from build123d import *

# Parameters (mm, degrees)
BOSS_EXTRUDE1_DEPTH = 38.1
SKETCH2_W           = 209.55
SKETCH2_H           = 38.1
BOSS_EXTRUDE2_DEPTH = 9.525
SKETCH3_W           = 20.32
SKETCH3_H           = 3.175
SKETCH3_H_2         = 6.35
SKETCH3_H_3         = 9.525
SKETCH3_H_4         = 12.7
SKETCH3_H_5         = 15.875
SKETCH3_H_6         = 19.05
SKETCH3_H_7         = 22.225
SKETCH3_H_8         = 25.4
CUT_EXTRUDE1_DEPTH  = 123.141181515
CHAMFER1_SIZE       = 25.4
CHAMFER2_SIZE       = 25.4
FILLET1_R           = 1.27
FILLET2_R           = 5.08


with BuildPart() as part:
    # Sketch1 → Boss-Extrude1 (new, symmetric)
    with BuildSketch(Plane.XY):
        Polygon((-105.823993484, 0), (103.726006516, 0), (103.726006516, 12.7), (-105.823993484, 25.4), align=None)
    extrude(amount=BOSS_EXTRUDE1_DEPTH, both=True)

    # Sketch2 → Boss-Extrude2 (add)
    with BuildSketch(Plane(origin=(0, 0, -38.1), x_dir=(-1, 0, 0), z_dir=(0, 0, -1))):
        with Locations((1.048993484, 19.05)):
            Rectangle(SKETCH2_W, SKETCH2_H)
    boss_extrude2 = extrude(amount=BOSS_EXTRUDE2_DEPTH)

    # Mirror1: Boss-Extrude2 across plane
    add(boss_extrude2.mirror(Plane.XY))

    # Sketch3 → Cut-Extrude1 (cut, through all)
    with BuildSketch(Plane.XZ):
        with Locations((-89.313993484, 0)):
            Rectangle(SKETCH3_W, SKETCH3_H)
        with Locations((-63.151993484, 0)):
            Rectangle(SKETCH3_W, SKETCH3_H_2)
        with Locations((-36.989993484, 0)):
            Rectangle(SKETCH3_W, SKETCH3_H_3)
        with Locations((-10.827993484, 0)):
            Rectangle(SKETCH3_W, SKETCH3_H_4)
        with Locations((15.334006516, 0)):
            Rectangle(SKETCH3_W, SKETCH3_H_5)
        with Locations((41.496006516, 0)):
            Rectangle(SKETCH3_W, SKETCH3_H_6)
        with Locations((67.658006516, 0)):
            Rectangle(SKETCH3_W, SKETCH3_H_7)
        with Locations((93.566006516, 0)):
            Rectangle(SKETCH3_W, SKETCH3_H_8)
    extrude(amount=-CUT_EXTRUDE1_DEPTH, mode=Mode.SUBTRACT)

    # Chamfer1
    # the kernel refuses this chamfer: 25.4 mm, written as the material it adds along each edge
    with BuildSketch(Plane(origin=(168.92711924, 8.748417411, 38.1), x_dir=(0.060472188242602316, 0.9977911060029382, 0.02749587661058647), z_dir=(-0.9981684966311909, 0.06049506040189036, 0))) as chamfer1_piece_1_section:
        Polygon((CHAMFER1_SIZE * 0.999621916911, CHAMFER1_SIZE * 0.0274958766106), (-CHAMFER1_SIZE * 0.0274958766106, CHAMFER1_SIZE * 0.999621916911), (0, 0), align=None)
    chamfer1_piece_1 = extrude(amount=340.575991525, mode=Mode.PRIVATE)
    chamfer1_piece_1 = split(chamfer1_piece_1, bisect_by=Plane(origin=(103.726006516, 21.644739683, 29.711789503), z_dir=(-1, 0, 0)), keep=Keep.TOP, mode=Mode.PRIVATE)
    chamfer1_piece_1 = split(chamfer1_piece_1, bisect_by=Plane(origin=(93.576497018, 21.644739683, 12.7), z_dir=(0, 0, 1)), keep=Keep.TOP, mode=Mode.PRIVATE)
    chamfer1_piece_1 = split(chamfer1_piece_1, bisect_by=Plane(origin=(83.406006516, 21.644739683, 29.711789503), z_dir=(1, 0, 0)), keep=Keep.TOP, mode=Mode.PRIVATE)
    chamfer1_piece_1 = split(chamfer1_piece_1, bisect_by=Plane(origin=(93.576497018, 38.1, 29.711789503), z_dir=(0, -1, 0)), keep=Keep.TOP, mode=Mode.PRIVATE)
    add(chamfer1_piece_1)
    with BuildSketch(Plane(origin=(168.92711924, 8.748417411, 38.1), x_dir=(0.060472188242602316, 0.9977911060029382, 0.02749587661058647), z_dir=(-0.9981684966311909, 0.06049506040189036, 0))) as chamfer1_piece_2_section:
        Polygon((CHAMFER1_SIZE * 0.999621916911, CHAMFER1_SIZE * 0.0274958766106), (-CHAMFER1_SIZE * 0.0274958766106, CHAMFER1_SIZE * 0.999621916911), (0, 0), align=None)
    chamfer1_piece_2 = extrude(amount=340.575991525, mode=Mode.PRIVATE)
    chamfer1_piece_2 = split(chamfer1_piece_2, bisect_by=Plane(origin=(-105.823993484, 26.508792165, 29.076634432), z_dir=(1, 0, 0)), keep=Keep.TOP, mode=Mode.PRIVATE)
    chamfer1_piece_2 = split(chamfer1_piece_2, bisect_by=Plane(origin=(-6.816832876, 26.508792165, 12.7), z_dir=(0, 0, 1)), keep=Keep.TOP, mode=Mode.PRIVATE)
    chamfer1_piece_2 = split(chamfer1_piece_2, bisect_by=Plane(origin=(83.406006516, 26.508792165, 29.076634432), z_dir=(-1, 0, 0)), keep=Keep.TOP, mode=Mode.PRIVATE)
    chamfer1_piece_2 = split(chamfer1_piece_2, bisect_by=Plane(origin=(-6.816832876, 38.1, 29.076634432), z_dir=(0, -1, 0)), keep=Keep.TOP, mode=Mode.PRIVATE)
    add(chamfer1_piece_2)

    # Chamfer2
    # the kernel refuses this chamfer: 25.4 mm, written as the material it adds along each edge
    with BuildSketch(Plane(origin=(168.92711924, 8.748417411, -38.1), x_dir=(0.060472188242602316, 0.9977911060029382, -0.02749587661058647), z_dir=(-0.9981684966311909, 0.06049506040189036, 0))) as chamfer2_piece_1_section:
        Polygon((CHAMFER2_SIZE * 0.999621916911, -CHAMFER2_SIZE * 0.0274958766106), (-CHAMFER2_SIZE * 0.0274958766106, -CHAMFER2_SIZE * 0.999621916911), (0, 0), align=None)
    chamfer2_piece_1 = extrude(amount=340.575991525, mode=Mode.PRIVATE)
    chamfer2_piece_1 = split(chamfer2_piece_1, bisect_by=Plane(origin=(93.576497018, 38.1, -29.711789503), z_dir=(0, -1, 0)), keep=Keep.TOP, mode=Mode.PRIVATE)
    chamfer2_piece_1 = split(chamfer2_piece_1, bisect_by=Plane(origin=(103.726006516, 21.644739683, -29.711789503), z_dir=(-1, 0, 0)), keep=Keep.TOP, mode=Mode.PRIVATE)
    chamfer2_piece_1 = split(chamfer2_piece_1, bisect_by=Plane(origin=(93.576497018, 21.644739683, -12.7), z_dir=(0, 0, -1)), keep=Keep.TOP, mode=Mode.PRIVATE)
    chamfer2_piece_1 = split(chamfer2_piece_1, bisect_by=Plane(origin=(83.406006516, 21.644739683, -29.711789503), z_dir=(1, 0, 0)), keep=Keep.TOP, mode=Mode.PRIVATE)
    add(chamfer2_piece_1)
    with BuildSketch(Plane(origin=(168.92711924, 8.748417411, -38.1), x_dir=(0.060472188242602316, 0.9977911060029382, -0.02749587661058647), z_dir=(-0.9981684966311909, 0.06049506040189036, 0))) as chamfer2_piece_2_section:
        Polygon((CHAMFER2_SIZE * 0.999621916911, -CHAMFER2_SIZE * 0.0274958766106), (-CHAMFER2_SIZE * 0.0274958766106, -CHAMFER2_SIZE * 0.999621916911), (0, 0), align=None)
    chamfer2_piece_2 = extrude(amount=340.575991525, mode=Mode.PRIVATE)
    chamfer2_piece_2 = split(chamfer2_piece_2, bisect_by=Plane(origin=(-105.823993484, 26.508792165, -29.076634432), z_dir=(1, 0, 0)), keep=Keep.TOP, mode=Mode.PRIVATE)
    chamfer2_piece_2 = split(chamfer2_piece_2, bisect_by=Plane(origin=(-6.816832876, 38.1, -29.076634432), z_dir=(0, -1, 0)), keep=Keep.TOP, mode=Mode.PRIVATE)
    chamfer2_piece_2 = split(chamfer2_piece_2, bisect_by=Plane(origin=(-6.816832876, 26.508792165, -12.7), z_dir=(0, 0, -1)), keep=Keep.TOP, mode=Mode.PRIVATE)
    chamfer2_piece_2 = split(chamfer2_piece_2, bisect_by=Plane(origin=(83.406006516, 26.508792165, -29.076634432), z_dir=(-1, 0, 0)), keep=Keep.TOP, mode=Mode.PRIVATE)
    add(chamfer2_piece_2)

    # Fillet1
    fillet1_edges = [part.edges().sort_by_distance(p)[0] for p in [
        (-20.987993484, 10.129212121, -6.35),
        (-20.987993484, 10.129212121, 6.35),
        (-0.667993484, 9.513454545, 6.35),
        (-0.667993484, 9.513454545, -6.35),
        (5.174006516, 9.336424242, -7.9375),
        (5.174006516, 9.336424242, 7.9375),
        (25.494006516, 8.720666667, 7.9375),
        (25.494006516, 8.720666667, -7.9375),
        (31.336006516, 8.543636364, -9.525),
        (31.336006516, 8.543636364, 9.525),
        (51.656006516, 7.927878788, 9.525),
        (51.656006516, 7.927878788, -9.525),
        (57.498006516, 7.750848485, -11.1125),
        (57.498006516, 7.750848485, 11.1125),
        (77.818006516, 7.135090909, 11.1125),
        (77.818006516, 7.135090909, -11.1125),
        (83.406006516, 6.965757576, -12.7),
        (83.406006516, 6.965757576, 12.7),
        (-99.473993484, 12.507575758, 1.5875),
        (-79.153993484, 11.891818182, 1.5875),
        (-79.153993484, 11.891818182, -1.5875),
        (-99.473993484, 12.507575758, -1.5875),
        (-73.311993484, 11.714787879, -3.175),
        (-73.311993484, 11.714787879, 3.175),
        (-52.991993484, 11.099030303, 3.175),
        (-52.991993484, 11.099030303, -3.175),
        (-47.149993484, 10.922, -4.7625),
        (-47.149993484, 10.922, 4.7625),
        (-26.829993484, 10.306242424, 4.7625),
        (-26.829993484, 10.306242424, -4.7625),
    ]]
    fillet(fillet1_edges, radius=FILLET1_R)

    # Fillet2
    fillet2_edges = [part.edges().sort_by_distance(p)[0] for p in [
        (-1.048993484, 0, -47.625),
        (-1.048993484, 38.1, -47.625),
        (-1.048993484, 38.1, 31.715109861),
        (-1.048993484, 38.1, -31.715109861),
        (-1.048993484, 38.1, 47.625),
        (-1.048993484, 0, 47.625),
    ]]
    fillet(fillet2_edges, radius=FILLET2_R)


solid = part.part
CAD build for the part. Positions are in the model's coordinates, mm. A direction names the side the tool comes from. Coordinates: 2 decimals unless noted, no trailing zeros. Order: outer loops, then holes, each group sorted by start corner. A loop starts at its lowest first (then second) coordinate and runs counter-clockwise, first axis right, second up.
Item 1: Band-saw the part on B-B on y = 9. Give the number of separate pieces and of enclosed holes in the cut face, plus the area to 3 significant figures.
Check sheet entries:
separate pieces: 1
enclosed holes: 7
area: 17,600 mm2
Item 2: Band-saw the part on C-C on z = 15. List the corners of the cut face in (x, y).
Check sheet entries:
outline: (-105.82, 0) - (103.73, 0) - (103.73, 15) - (-105.82, 27.7) - close
Item 3: Drill centre lines: L1, parallel to Z at x = -82, y = 7.5 (1 decimal); L2, parallel to Y at x = -47, z = 6; L3, parallel to Z at x = 5.5, y = 24 (3 decimals). Where is each one in solid material? Low to high.
Check sheet entries:
L1: z = -47.6 to -1.6, 1.6 to 47.6
L2: y = 0 to 21.83
L3: z = -47.625 to -18.037, 18.037 to 47.625
Item 4: Pin check, flat tips, straight feed: pin 1 Ø1.9 at (y, z) = (7, 0) entering from +X; pin 2 Ø11 at (x, y) = (91.5, 3.5) entering from +Z (3 decimals). Stop position of each tip, or through.
Check sheet entries:
pin 1: stops at x = 83.41
pin 2: stops at z = 47.625
Item 5: Two-plate mould, pull along X, no slides. Class faces 4 (the face through (-2.52, 1.45, -46.1)), 5 (the face through (-20.988, 10, 0)), 6 (the face through (103.726, 15, 34)): +X half, -X half, draft (parallel to the pull), parting line (faces both ways), or undercut.
Check sheet entries:
face 4: draft
face 5: undercut
face 6: +X half
Item 6: 3-axis set-ups, long thin cutter, end or side, ignore diameter. For faces 1 (the face through (94, 7, 12.7)), 2 (the face through (25.494, 9, 0)), 3 (the face through (24.014, 26.995, -22.147)): which of +Z, -Z, +X, -X, +Y, -Y reach the whole face in a straight line?
Check sheet entries:
face 1: +X, +Y, -Y
face 2: +Y, -Y
face 3: +X, +Y
Item 7: Band-saw the part on A-A on y = 29.5. List the corners of the cut face in (x, z) (1 decimal).
Check sheet entries:
outline: (-105.8, -47.6) - (103.7, -47.6) - (103.7, -29.5) - (-105.8, -16.8) - close; (-105.8, 16.8) - (103.7, 29.5) - (103.7, 47.6) - (-105.8, 47.6) - close
